Answer from the drawing. Dimensions are ordinates in mm from the lowest x, y and z of the part. A direction names the side the tool comes from. Coordinates: 2 decimals unless noted, no trailing zeros. Loops run counter-clockwise (first coordinate to the right, second up) from the corner with the lowest first, then second, coordinate; pieces in that order, holes last. Notation, with made-up numbers: (-35, -19.5) -> (17, -19.5) arc R6 ccw to (17, -8.5) -> close; hole circle Ø5 at (59.5, -25). An arc over 180 degrees is marked (long way). Answer as CSV lines item,"result".
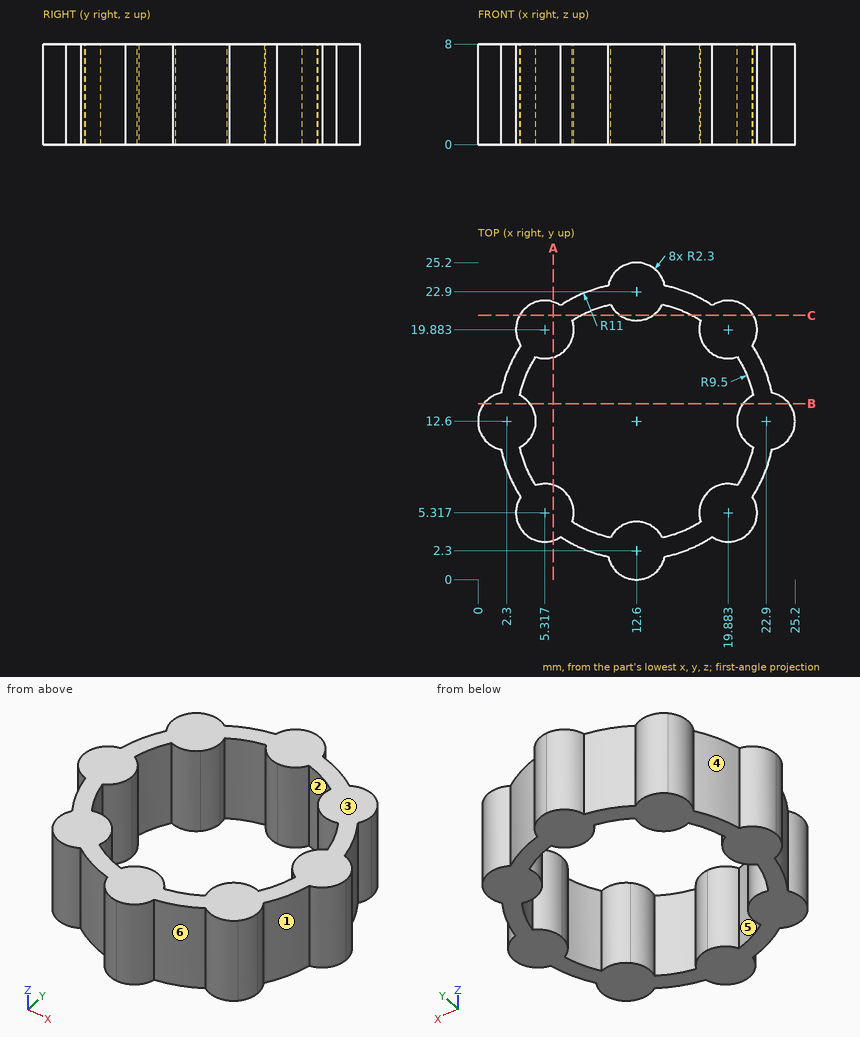
(1) A cutting plane is placed at B-B, the plane y = 14. Write down the section's boundary in (x, z) (1 decimal).
Computed values:
outline,"(0.5, 0) -> (4.1, 0) -> (4.1, 8) -> (0.5, 8) -> close; (21.1, 0) -> (24.7, 0) -> (24.7, 8) -> (21.1, 8) -> close"
(2) For a pull along X with two mould halves and no side action, classify the marked faces 1, 2 and 3 as pulls with the +X half, pulls with the -X half, needs draft (parallel to the pull), parting line crosses it, or undercut.
Computed values:
face 1,"pulls with the +X half"
face 2,"undercut"
face 3,"needs draft"
(3) Flat-ended cylindrical pins translate along their axes: pin 1 Ø1.5 at (x, z) = (22.5, 2.5) entering from -Y; pin 2 Ø4 at (x, z) = (17.5, 2) entering from -Y. Find the tip coordinate at first contact, or state that the pin passes through.
Computed values:
pin 1,"y = 3.97"
pin 2,"y = 1.99"
(4) A cutting plane is placed at A-A, the plane x = 6. Write down the section's boundary in (y, z).
Computed values:
outline,"(3.12, 0) -> (7.51, 0) -> (7.51, 8) -> (3.12, 8) -> close; (17.69, 0) -> (22.08, 0) -> (22.08, 8) -> (17.69, 8) -> close"
(5) Consider line 1 along Y through (x, z) = (20, 5.25); line 2 along X through (y, z) = (12.5, 4); line 3 along X through (y, z) = (3.25, 1.75) (1 decimal). Determine where each line is inside the solid, lowest interval first.
Computed values:
line 1,"3.02 to 7.61, 17.59 to 22.18"
line 2,"0 to 4.6, 20.6 to 25.2"
line 3,"4.3 to 6.3, 6.8 to 18.4, 18.9 to 20.9"
(6) A cutting plane is placed at C-C, the plane y = 21. Write down the section's boundary in (x, z).
Computed values:
outline,"(3.31, 0) -> (8.16, 0) -> (8.16, 8) -> (3.31, 8) -> close; (11.3, 0) -> (13.9, 0) -> (13.9, 8) -> (11.3, 8) -> close; (17.04, 0) -> (21.89, 0) -> (21.89, 8) -> (17.04, 8) -> close"
(7) Which of the six approach directions +Z, -Z, +X, -X, +Y, -Y give full straight-line access (tool end or side, diameter ignored) to the marked faces 4, 5 and 6?
Computed values:
face 4,"+Z, -Z, -X"
face 5,"+Z, -Z"
face 6,"+Z, -Z, -Y"
